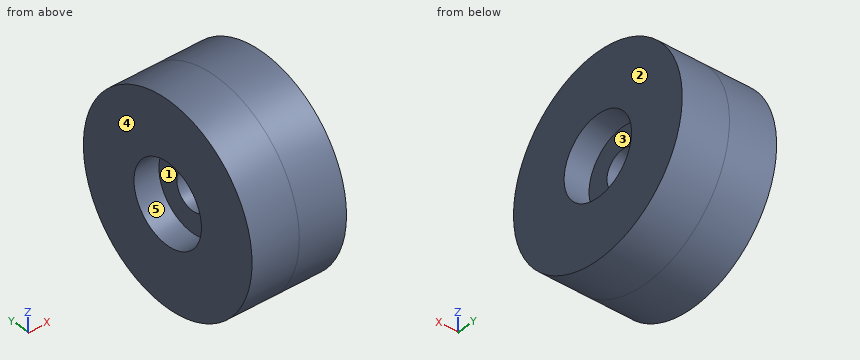
from build123d import *


with BuildPart() as part:
    # Sketch1 → Revolve1 (revolve)
    with BuildSketch(Plane.XY):
        Polygon((0, -25), (0, -133.35), (-63.5, -133.35), (-63.5, -53.35), (-30, -53.35), (-30, -25), align=None)
    revolve1 = revolve(axis=Axis((-62.857142857, 0, 0), (1, 0, 0)))

    # Mirror1: Revolve1 across plane
    add(revolve1.mirror(Plane(origin=(0, 0, 0), x_dir=(0, 0, 1), z_dir=(1, 0, 0))))


solid = part.part
Geometry check sheet. Reference: the model listing, model coordinates, mm. Face numbers are marked on the shaded views. A direction names the side the tool comes from. Round coordinates to 2 decimals unless told otherwise and drop trailing zeros. Order: outer loops, then holes, each group sorted by start corner. A loop starts at its lowest first (then second) coordinate and runs counter-clockwise, first axis right, second up. Notation, with made-up numbers: M 30.5,28 L 82.5,28 A14 ccw 82.5,54 Z; hole C 48,-10.75 d7. An arc over 180 degrees is marked long. Answer in a Markdown table with one row per item.
(1) Sectioned sample at A-A, the plane z = 0. Record the cut outline in (x, y).
Responses:
| item | result |
|---|---|
| outline | M -63.5,-133.35 L 63.5,-133.35 L 63.5,-53.35 L 30,-53.35 L 30,-25 L -30,-25 L -30,-53.35 L -63.5,-53.35 Z; M -63.5,53.35 L -30,53.35 L -30,25 L 30,25 L 30,53.35 L 63.5,53.35 L 63.5,133.35 L -63.5,133.35 Z |
(2) Scan lines: probe 1 along Z at (x, y) = (-17.5, 0); probe 2 along Y at (x, z) = (38, 0); probe 3 along X at (y, z) = (49.5, 15.5). Record each from-to range of solid material in increasing order. Write a range as from..to.
Responses:
| item | result |
|---|---|
| probe 1 | z = -133.35..-25, 25..133.35 |
| probe 2 | y = -133.35..-53.35, 53.35..133.35 |
| probe 3 | x = -30..30 |
(3) Tool access check on the marked faces 3, 4 and 5. Record the directions out of +Z, -Z, +X, -X, +Y, -Y that give a thin tool (end or side, any length) a straight path to the whole face; none if there is none.
Responses:
| item | result |
|---|---|
| face 3 | +X |
| face 4 | +Z, -Z, -X, +Y, -Y |
| face 5 | -X |
(4) Sectioned sample at C-C, the plane x = -52. Record the cut outline in (y, z), and give its area (3 significant figures).
Responses:
| item | result |
|---|---|
| outline | C 0,0 d266.7; hole C 0,0 d106.7 |
| area | 46,900 mm² |
(5) Sectioned sample at D-D, the plane z = 39.5. Record the cut outline in (x, y), and give its area (3 significant figures).
Responses:
| item | result |
|---|---|
| outline | M -63.5,-127.37 L 63.5,-127.37 L 63.5,-35.86 L 30,-35.86 L 30,35.86 L 63.5,35.86 L 63.5,127.37 L -63.5,127.37 L -63.5,35.86 L -30,35.86 L -30,-35.86 L -63.5,-35.86 Z |
| area | 27,500 mm² |
(6) Go/stop test with flat-tipped pins: P1, Ø12, axis at y = -101.5, z = -97, coming from the +X side; P2, Ø1.5, axis at y = -23, z = -11.5, coming from the +X side; P3, Ø8, axis at x = -36, y = 68.5, coming from the +Z side; P4, Ø8, axis at x = -23.5, y = -60.5, coming from the -Z side. Record where each tip stops, or that it passes through.
Responses:
| item | result |
|---|---|
| P1 | passes through |
| P2 | stops at x = 30 |
| P3 | stops at z = 116.71 |
| P4 | stops at z = -120.79 |
(7) Draft check along Z on the marked faces 1 and 2. Enter one of: released by +Z, released by -Z, zero draft, split by the parting line, or undercut.
Responses:
| item | result |
|---|---|
| face 1 | undercut |
| face 2 | zero draft |
